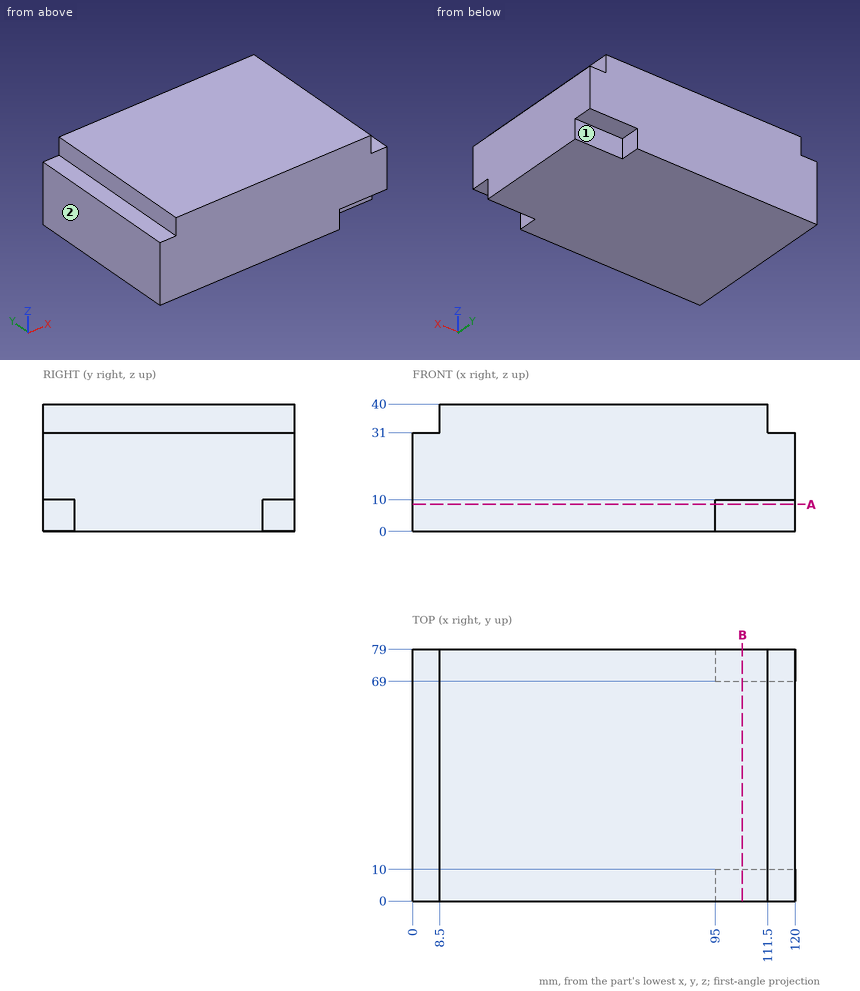
Geometry check sheet. Reference: drawing and pictorial views, mm from the part's lowest x, y, z. A direction names the side the tool comes from. Round coordinates to 2 decimals unless told otherwise and drop trailing zeros. Loops run counter-clockwise (first coordinate to the right, second up) from the corner with the lowest first, then second, coordinate; pieces in that order, holes last. Notation, with made-up numbers: (78, 50.5) -> (98, 50.5) arc R13 cw to (98, 64.5) -> close; hole circle Ø8 at (75.5, 24). An arc over 180 degrees is marked (long way). Use a Markdown table: item, result.
(1) Set-up check for the marked faces 1 and 2: record each of +Z, -Z, +X, -X, +Y, -Y from which the full face is reachable in a straight line by a thin tool's end or side.
Calculated:
| item | result |
|---|---|
| face 1 | -Z, +X, +Y |
| face 2 | +Z, -Z, -X, +Y, -Y |
(2) Sectioned sample at B-B (x = 103.5). Enter the section's corners in (y, z).
Calculated:
| item | result |
|---|---|
| outline | (0, 10) -> (10, 10) -> (10, 0) -> (69, 0) -> (69, 10) -> (79, 10) -> (79, 40) -> (0, 40) -> close |
(3) Go/stop test with flat-tipped pins: P1, Ø5, axis at y = 5, z = 4.5, coming from the +X side; P2, Ø3, axis at x = 112, y = 6.5, coming from the -Z side; P3, Ø4.5, axis at y = 21.5, z = 34.5, coming from the +X side. Record where each tip stops, or that it passes through.
Calculated:
| item | result |
|---|---|
| P1 | x = 95 |
| P2 | z = 10 |
| P3 | x = 111.5 |
(4) Sectioned sample at A-A (z = 8.5). Enter the section's corners in (x, y).
Calculated:
| item | result |
|---|---|
| outline | (0, 0) -> (95, 0) -> (95, 10) -> (120, 10) -> (120, 69) -> (95, 69) -> (95, 79) -> (0, 79) -> close |
(5) Scan lines: probe 1 along X at (y, z) = (34.5, 38.5); probe 2 along X at (y, z) = (9, 8). Record each from-to range of solid material in increasing order.
Calculated:
| item | result |
|---|---|
| probe 1 | 8.5 to 111.5 |
| probe 2 | 0 to 95 |
